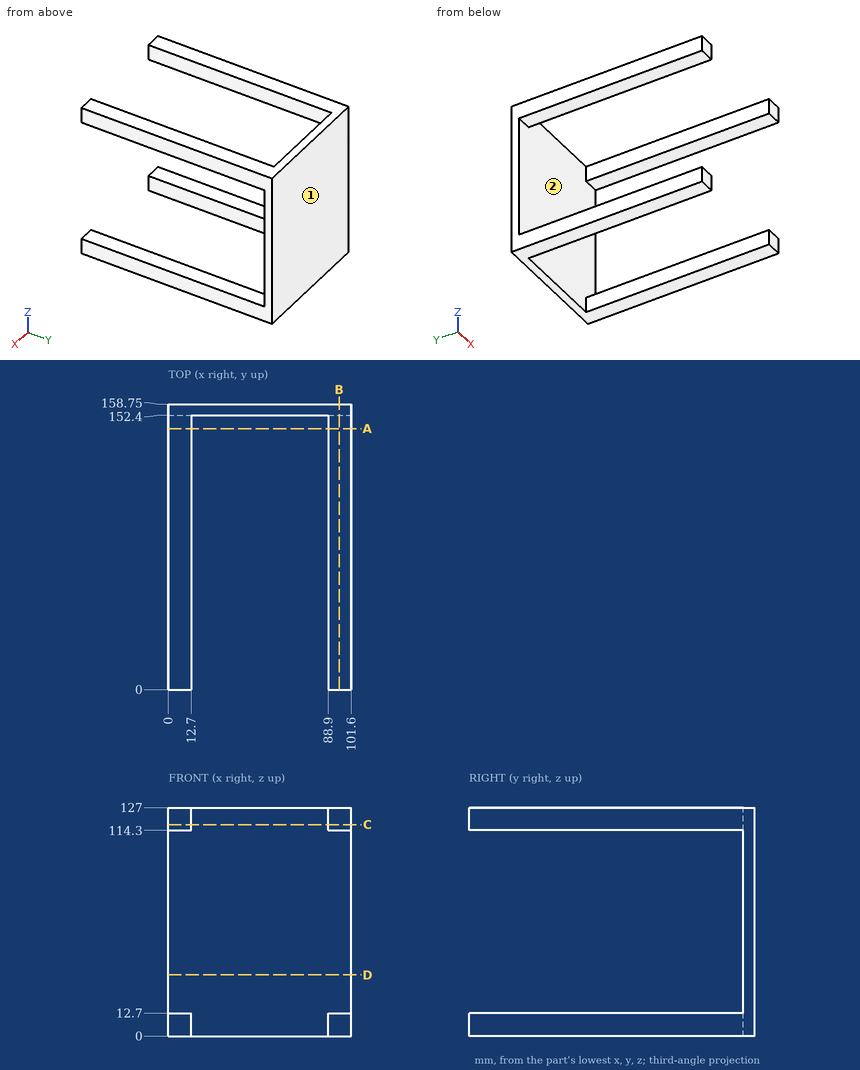
Print and shaded views of the part. All mm, measured from the part's lowest x, y and z. Give positions to 0.01 mm unless a question says otherwise; leave off trailing zeros. Loops run counter-clockwise (first coordinate to the right, second up) from the corner with the lowest first, then second, coordinate; pieces in that order, holes last.
1) Saw through at A-A (y = 145). Write the cut outline in (x, z), plus the area to 3 significant figures.
2) Saw through at C-C (z = 117.5). Write the cut outline in (x, y), plus the area to 3 significant figures.
3) Wall check: line 1 (Z direction, x = 6, y = 14); line 2 (Y direction, x = 35, z = 51.5). Give the ranges that are in metal, low to high.
4) Pull direction Z, two halves, no side cores. Call the marked faces 1 and 2: +Z half, -Z half, draft (parallel to the pull), parting line (faces both ways), or undercut.
5) Saw through at D-D (z = 34). Write the cut outline in (x, y), plus the area to 3 significant figures.
6) Saw through at B-B (x = 95). Write the cut outline in (y, z), plus the area to 3 significant figures.
7) Flat gauge pins, fed straight in: pin 1 Ø12 at (x, y) = (77.5, 112) entering from +Z; pin 2 Ø4 at (x, z) = (22.5, 35.5) entering from -Y; pin 3 Ø6.5 at (x, y) = (92.5, 62.5) entering from -Z. Where does each tip first touch, or does it go through?
Answer block:
1. outline: (0, 0) - (12.7, 0) - (12.7, 12.7) - (0, 12.7) - close; (0, 114.3) - (12.7, 114.3) - (12.7, 127) - (0, 127) - close; (88.9, 0) - (101.6, 0) - (101.6, 12.7) - (88.9, 12.7) - close; (88.9, 114.3) - (101.6, 114.3) - (101.6, 127) - (88.9, 127) - close
1. area: 645 mm2
2. outline: (0, 0) - (12.7, 0) - (12.7, 152.4) - (88.9, 152.4) - (88.9, 0) - (101.6, 0) - (101.6, 158.75) - (0, 158.75) - close
2. area: 4,520 mm2
3. line 1: z = 0 to 12.7, 114.3 to 127
3. line 2: y = 152.4 to 158.75
4. face 1: draft
4. face 2: undercut
5. outline: (0, 152.4) - (101.6, 152.4) - (101.6, 158.75) - (0, 158.75) - close
5. area: 645 mm2
6. outline: (0, 0) - (158.75, 0) - (158.75, 127) - (0, 127) - (0, 114.3) - (152.4, 114.3) - (152.4, 12.7) - (0, 12.7) - close
6. area: 4,680 mm2
7. pin 1: passes through
7. pin 2: stops at y = 152.4
7. pin 3: stops at z = 0
